Geometry: final body of the model. Coordinates: model frame, mm. A direction names the side the tool comes from. Coordinates: 2 decimals unless noted, no trailing zeros. Loops run counter-clockwise (first coordinate to the right, second up) from the corner with the lowest first, then second, coordinate; pieces in that order, holes last. Notation, with made-up numbers: (-19.75, 74) - (-5.75, 74) arc R10 cw to (-5.75, 80) - close; hole circle Ø3 at (57.25, 39.5). An arc over 180 degrees is marked (long way). Return JSON: item names as keys, results as strings.
from build123d import *

# Parameters (mm, degrees)
F0_W     = 250
F0_H     = 150
F1_DEPTH = 30
F2_R     = 7.0739
F3_DEPTH = 40
F4_SIZE  = 3


with BuildPart() as f1:
    # F0 (on Top) → F1 (new body)
    with BuildSketch(Plane.XY):
        with Locations((17.895456, -6.518978)):
            Rectangle(F0_W, F0_H)
    extrude(amount=-F1_DEPTH)

    # F2 (on face) → F3 (join)
    with BuildSketch(Plane(origin=(0, 0, -30), x_dir=(1, 0, 0), z_dir=(0, 0, -1))):
        with Locations((-80.976687, 64.177193)):
            Circle(F2_R)
        with Locations((121.452317, 64.177193)):
            Circle(F2_R)
        with Locations((121.452317, -50.98886)):
            Circle(F2_R)
        with Locations((-80.976687, -50.98886)):
            Circle(F2_R)
    extrude(amount=F3_DEPTH)

    # F4
    f4_edges = [f1.edges().sort_by_distance(p)[0] for p in [
        (-107.104544, 68.481022, -15),
        (142.895456, 68.481022, -15),
        (142.895456, -81.518978, -15),
        (-107.104544, -81.518978, -15),
    ]]
    chamfer(f4_edges, length=F4_SIZE)


solid = f1.part
Item 1: Section query C-C, the plane z = -50. Return loops of the section in (x, y).
Worked out:
{"outline": "circle Ø14.15 at (-80.98, -64.18); circle Ø14.15 at (-80.98, 50.99); circle Ø14.15 at (121.45, -64.18); circle Ø14.15 at (121.45, 50.99)"}
Item 2: Ray query, probe 1 along Z at (x, y) = (47, -28.5); probe 2 along Y at (x, z) = (-83, -65); probe 3 along Y at (x, z) = (-87.5, -40) (3 decimals). Return the intervals inside material, ascending. Write a range as from..to.
Worked out:
{"probe 1": "-30..0", "probe 2": "-70.96..-57.4, 44.21..57.77", "probe 3": "-66.913..-61.441, 48.253..53.725"}
Item 3: Section query A-A, the plane x = -20. Return loops of the section in (y, z), and give its area (3 significant figures).
Worked out:
{"outline": "(-81.52, -30) - (68.48, -30) - (68.48, 0) - (-81.52, 0) - close", "area": "4,500 mm^2"}
Item 4: Mould query, pull axis X, two halves, no side actions, for faces 1 (the face through (-86.59, -59.87, -49.72)), 2 (the face through (121, 51, -70)), 3 (the face through (142.895, -8, -15)). Classes: +X half, -X half, draft (parallel to the pull), parting line (faces both ways), or undercut.
Worked out:
{"face 1": "undercut", "face 2": "draft", "face 3": "+X half"}
Item 5: First-contact query: pin 1 Ø1 at (x, y) = (24, 13.5) entering from -Z. Flat tip, straight axial feed; report the tip coordinate or a pass-through.
Worked out:
{"pin 1": "z = -30"}
Item 6: Section query B-B, the plane y = 32. Return loops of the section in (x, z), and give its area (3 significant figures).
Worked out:
{"outline": "(-107.1, -30) - (142.9, -30) - (142.9, 0) - (-107.1, 0) - close", "area": "7,500 mm^2"}
Item 7: Reachability of faces 4 (the face through (127.987, 53.698, -49.72)), 5 (the face through (-107.105, -8, -15)) from +Z, -Z, +X, -X, +Y, -Y: full face, straight path, thin tool, end or side. Return the list, or none.
Worked out:
{"face 4": "-Z", "face 5": "+Z, -Z, -X, +Y, -Y"}
